Can you work these out from the model? Positions are in its coordinate system, mm. A direction names the side the tool comes from. Round coordinates to 2 decimals unless told otherwise and drop trailing zeros. Order: outer loops, then holes, each group sorted by start corner. A loop starts at its lowest first (then second) coordinate and runs counter-clockwise, first axis right, second up.
from build123d import *

# Parameters (mm, degrees)
FL_CHE_START                         = -6
FL_CHE_VERSCHIEBEN1_2_OUTLINE_R      = 1.25
FL_CHE_VERSCHIEBEN1_2_DEPTH          = 12
FL_CHE_START_2                       = 1.833034949
FL_CHE_VERSCHIEBEN1_3_OUTLINE_R      = 0.8
FL_CHE_VERSCHIEBEN1_3_DEPTH          = 4.166965051
SCHNITT_LINEAR_AUSTRAGEN1_DEPTH      = 20
SCHNITT_LINEAR_AUSTRAGEN1_DEPTH_BACK = 4.5
SKIZZE1_R                            = 4.5
SKIZZE2_R                            = 4
AUFSATZ_LINEAR_AUSTRAGEN1_DEPTH      = 15
SCHNITT_LINEAR_START                 = -1
SKIZZE3_R                            = 4.5
SKIZZE3_R_2                          = 3
SCHNITT_LINEAR_AUSTRAGEN2_DEPTH      = 6
FASE1_SIZE                           = 0.5
SCHNITT_LINEAR_AUSTRAGEN3_DEPTH      = 10
SCHNITT_LINEAR_AUSTRAGEN3_DEPTH_BACK = 10
SKIZZE5_R                            = 0.8


with BuildPart() as part:
    # Fläche verschieben1: read off the stored shape, not the designer's step
    # Fläche verschieben1 outline → Fläche verschieben1 (revolve)
    with BuildSketch(Plane.YX):
        with BuildLine():
            ThreePointArc((1.75, 26.8), (1.808578644, 26.941421356), (1.95, 27))
            Line((1.95, 27), (2, 27))
            Line((2, 27), (2, 33.85))
            Line((2, 33.85), (1.85, 34))
            Line((1.85, 34), (0, 34))
            Line((0, 34), (0, 10.18519763))
            Line((0, 10.18519763), (2, 8.983476392))
            Line((2, 8.983476392), (2, 0))
            Line((2, 0), (4.5, 0))
            Line((4.5, 0), (4.5, 20))
            Line((4.5, 20), (3, 20))
            Line((3, 20), (3, 26))
            Line((3, 26), (1.95, 26))
            ThreePointArc((1.95, 26), (1.808578644, 26.058578644), (1.75, 26.2))
            Line((1.75, 26.2), (1.75, 26.8))
        make_face()
    revolve(axis=Axis((0, 0, 0), (1, 0, 0)))

    # Fl_che verschieben1 2 outline → Fl_che verschieben1 2 (cut)
    with BuildSketch(Plane.XY.offset(FL_CHE_START)):
        with Locations((17, 0)):
            Circle(FL_CHE_VERSCHIEBEN1_2_OUTLINE_R)
    extrude(amount=FL_CHE_VERSCHIEBEN1_2_DEPTH, mode=Mode.SUBTRACT)

    # Fl_che verschieben1 3 outline → Fl_che verschieben1 3 (cut)
    with BuildSketch(Plane.XY.offset(FL_CHE_START_2)):
        with Locations((7, 0)):
            Circle(FL_CHE_VERSCHIEBEN1_3_OUTLINE_R)
    extrude(amount=FL_CHE_VERSCHIEBEN1_3_DEPTH, mode=Mode.SUBTRACT)

    # Skizze1 → Schnitt-Linear austragen1 (cut, two sides: drawn at the far end of the back side and taken through both)
    with BuildSketch(Plane(origin=(20, 0, 0), x_dir=(0, 0, -1), z_dir=(1, 0, 0)).offset(-SCHNITT_LINEAR_AUSTRAGEN1_DEPTH_BACK)):
        with Locations(Location((0, 0, 0), (0, 0, 180))):
            Circle(SKIZZE1_R)
    extrude(amount=SCHNITT_LINEAR_AUSTRAGEN1_DEPTH + SCHNITT_LINEAR_AUSTRAGEN1_DEPTH_BACK, mode=Mode.SUBTRACT)

    # Skizze2 → Aufsatz-Linear austragen1 (add)
    with BuildSketch(Plane(origin=(15.5, 0, 0), x_dir=(0, 0, -1), z_dir=(1, 0, 0))):
        Circle(SKIZZE2_R)
    extrude(amount=AUFSATZ_LINEAR_AUSTRAGEN1_DEPTH)

    # Skizze3 → Schnitt-Linear austragen2 (cut)
    with BuildSketch(Plane(origin=(15.5, 0, 0), x_dir=(0, 0, -1), z_dir=(1, 0, 0)).offset(SCHNITT_LINEAR_START)):
        with Locations(Location((0, 0, 0), (0, 0, 180))):
            Circle(SKIZZE3_R)
        Circle(SKIZZE3_R_2, mode=Mode.SUBTRACT)
    extrude(amount=-SCHNITT_LINEAR_AUSTRAGEN2_DEPTH, mode=Mode.SUBTRACT)

    # Skizze4 → Schnitt-Rotation1 (revolve, cut)
    with BuildSketch(Plane(origin=(0, 0, 0), x_dir=(1, 0, 0), z_dir=(0, 1, 0)), mode=Mode.PRIVATE) as schnitt_rotation1_sk:
        Polygon((18.5, 4), (18.5, 3.2), (21.5, 3.2), (21.7, 4), align=None)
    revolve(schnitt_rotation1_sk.sketch.rotate(Axis((17.168940626, 0, 0), (1, 0, 0)), 180), axis=Axis((17.168940626, 0, 0), (1, 0, 0)), mode=Mode.SUBTRACT)

    # Fase1
    fase1_edges = [part.edges().sort_by_distance(p)[0] for p in [
        (30.5, 0, 4),
    ]]
    chamfer(fase1_edges, length=FASE1_SIZE)

    # Skizze5 → Schnitt-Linear austragen3 (cut, two sides: drawn at the far end of the back side and taken through both)
    with BuildSketch(Plane.XY.offset(-SCHNITT_LINEAR_AUSTRAGEN3_DEPTH_BACK)):
        with Locations(Location((11.3, 0, 0), (0, 0, 180))):
            Circle(SKIZZE5_R)
    extrude(amount=SCHNITT_LINEAR_AUSTRAGEN3_DEPTH + SCHNITT_LINEAR_AUSTRAGEN3_DEPTH_BACK, mode=Mode.SUBTRACT)


solid = part.part
(1) I want a section at D-D, the plane x = 20. List the corners of the cut face in (y, z) for me.
(2) I want a section at C-C, the plane x = 11.3. List the corners of the cut face in (y, z) for me.
(3) Please list where these lines run through material, in increasing order: probe 1 along X at (y, z) = (3.75, -2); probe 2 along X at (y, z) = (-0.75, -3.5); probe 3 along X at (y, z) = (1.25, 3.5).
(4) If we mould it in two halves opening along Y, with no side actions, what happens to faces 1 (the face through (15.007, 4.292, 1.352)), 2 (the face through (0, -1, -2)), 3 (the face through (9.976, -0.075, -0.339))? For each: pulls with the +Y half, pulls with the -Y half, needs draft (parallel to the pull), parting line crosses it, or undercut.
(5) I want a section at A-A, the plane x = 4. List the corners of the cut face in (y, z) for me.
(6) I want a section at B-B, the plane x = 24.5. List the corners of the cut face in (y, z) for me, plus the area to 3 significant figures.
(7) I'm going to push flat-ended pins straight in: pin 1 Ø1.5 at (x, y) = (6.5, 3.5) entering from -Z; pin 2 Ø5 at (x, y) = (15.5, 3.5) entering from +Z; pin 3 Ø2.5 at (y, z) = (0, 0) entering from -X. Where does each tip first touch, or does it pass through?
(8) On a 3-axis mill with a long thin cutter (end or side, diameter ignored), from which of +Z, -Z, +X, -X, +Y, -Y can I reach the whole of each face in a straight line? I mean faces 4 (the face through (16.979, -3.905, 0.867)), 5 (the face through (11.54, -1.15, -2.77)), 6 (the face through (4, 0, -2)). Say none if no direction works.
Ans:
1. outline: circle Ø6.4 at (0, 0)
2. outline: (-0.8, -2.89) - (-0.8, 2.89) arc R3 ccw to start; (0.8, -2.89) arc R3 ccw to (0.8, 2.89) - close
3. probe 1: x = 0 to 8.5, 14.5 to 15.5
3. probe 2: x = 0 to 8.5, 14.5 to 18.5, 21.59 to 30.42
3. probe 3: x = 0 to 8.5, 14.5 to 18.5, 21.63 to 30.28
4. face 1: parting line crosses it
4. face 2: needs draft
4. face 3: undercut
5. outline: circle Ø9 at (0, 0); hole circle Ø4 at (0, 0)
6. outline: circle Ø8 at (0, 0)
6. area: 50.3 mm2
7. pin 1: stops at z = -3.56
7. pin 2: stops at z = 4.39
7. pin 3: stops at x = 9.43
8. face 4: +X
8. face 5: none
8. face 6: -X
